Source: CAD feature listing. Evaluate the final solid. Frame: model axes, mm. A direction names the side the tool comes from. Give positions to 0.01 mm unless a question says otherwise; leave off trailing zeros. Loops run counter-clockwise (first coordinate to the right, second up) from the corner with the lowest first, then second, coordinate; pieces in that order, holes last. Notation, with made-up numbers: (-18, -27) -> (34, -27) arc R32 ccw to (34, 9) -> close; hole circle Ø8 at (7.5, 19). An arc over 180 degrees is marked (long way). Return JSON: item names as keys, results as strings. Group by question number.
```python
from build123d import *

# Parameters (mm, degrees)
SKETCH1_R               = 7.5
SKETCH1_R_2             = 2.75
SKETCH1_R_3             = 2.5
BOSS_EXTRUDE1_DEPTH     = 6
CUT_EXTRUDE1_DEPTH      = 70.758959998
CUT_EXTRUDE1_DEPTH_BACK = 70.758959998


with BuildPart() as part:
    # Sketch1 → Boss-Extrude1 (new body)
    # profile 1 of 7: a face of its own
    with BuildSketch(Plane(origin=(0, 0, 0), x_dir=(1, 0, 0), z_dir=(0, 1, 0))):
        with Locations((-52.25, 15.75)):
            Circle(SKETCH1_R)
        with Locations(Location((-52.25, 15.75, 0), (0, 0, 270))):
            Circle(SKETCH1_R_2, mode=Mode.SUBTRACT)
    # profile 2 of 7: a face of its own
    with BuildSketch(Plane(origin=(0, 0, 0), x_dir=(1, 0, 0), z_dir=(0, 1, 0))):
        with BuildLine():
            ThreePointArc((-44.75, 15.75), (-52.25, 8.25), (-59.75, 15.75))
            Line((-59.75, 15.75), (-59.75, -15.75))
            ThreePointArc((-59.75, -15.75), (-52.25, -8.25), (-44.75, -15.75))
            ThreePointArc((-44.75, -15.75), (-48.076702535, -21.981660154), (-55.105623539, -22.685085739))
            Line((-55.105623539, -22.685085739), (-25.355623539, -34.935085739))
            ThreePointArc((-25.355623539, -34.935085739), (-26.673297465, -21.768339846), (-15, -28))
            ThreePointArc((-15, -28), (-17.196699141, -33.303300859), (-22.5, -35.5))
            Line((-22.5, -35.5), (22.5, -35.5))
            ThreePointArc((22.5, -35.5), (17.196699141, -22.696699141), (30, -28))
            Line((30, -28), (30, 28))
            ThreePointArc((30, 28), (17.196699141, 22.696699141), (22.5, 35.5))
            Line((22.5, 35.5), (-22.5, 35.5))
            ThreePointArc((-22.5, 35.5), (-17.196699141, 33.303300859), (-15, 28))
            ThreePointArc((-15, 28), (-26.673297465, 21.768339846), (-25.355623539, 34.935085739))
            Line((-25.355623539, 34.935085739), (-55.105623539, 22.685085739))
            ThreePointArc((-55.105623539, 22.685085739), (-48.076702535, 21.981660154), (-44.75, 15.75))
        make_face()
        with Locations(Location((1.25, -15.75, 0), (0, 0, 270))):
            Circle(SKETCH1_R_2, mode=Mode.SUBTRACT)
        with Locations(Location((1.25, 15.75, 0), (0, 0, 270))):
            Circle(SKETCH1_R_2, mode=Mode.SUBTRACT)
    # profile 3 of 7: a face of its own
    with BuildSketch(Plane(origin=(0, 0, 0), x_dir=(1, 0, 0), z_dir=(0, 1, 0))):
        with Locations((-52.25, -15.75)):
            Circle(SKETCH1_R)
        with Locations(Location((-52.25, -15.75, 0), (0, 0, 270))):
            Circle(SKETCH1_R_2, mode=Mode.SUBTRACT)
    # profile 4 of 7: a face of its own
    with BuildSketch(Plane(origin=(0, 0, 0), x_dir=(1, 0, 0), z_dir=(0, 1, 0))):
        with Locations((-22.5, -28)):
            Circle(SKETCH1_R)
        with Locations(Location((-22.5, -23.5, 0), (0, 0, 270))):
            Circle(SKETCH1_R_3, mode=Mode.SUBTRACT)
    # profile 5 of 7: a face of its own
    with BuildSketch(Plane(origin=(0, 0, 0), x_dir=(1, 0, 0), z_dir=(0, 1, 0))):
        with Locations((22.5, -28)):
            Circle(SKETCH1_R)
        with Locations(Location((22.5, -23.5, 0), (0, 0, 270))):
            Circle(SKETCH1_R_3, mode=Mode.SUBTRACT)
    # profile 6 of 7: a face of its own
    with BuildSketch(Plane(origin=(0, 0, 0), x_dir=(1, 0, 0), z_dir=(0, 1, 0))):
        with Locations((22.5, 28)):
            Circle(SKETCH1_R)
        with Locations(Location((22.5, 23.5, 0), (0, 0, 270))):
            Circle(SKETCH1_R_3, mode=Mode.SUBTRACT)
    # profile 7 of 7: a face of its own
    with BuildSketch(Plane(origin=(0, 0, 0), x_dir=(1, 0, 0), z_dir=(0, 1, 0))):
        with Locations((-22.5, 28)):
            Circle(SKETCH1_R)
        with Locations(Location((-22.5, 23.5, 0), (0, 0, 270))):
            Circle(SKETCH1_R_3, mode=Mode.SUBTRACT)
    extrude(amount=BOSS_EXTRUDE1_DEPTH)

    # Sketch2 → Cut-Extrude1 (cut, two sides: drawn at the far end of the back side and taken through both)
    with BuildSketch(Plane(origin=(0, 6, 0), x_dir=(1, 0, 0), z_dir=(0, 1, 0)).offset(-CUT_EXTRUDE1_DEPTH_BACK)):
        Polygon((-52.25, 11.131197846), (-48.25, 13.440598923), (-48.25, 18.059401077), (-52.25, 20.368802154), (-56.25, 18.059401077), (-56.25, 13.440598923), align=None)
        Polygon((-52.25, -11.131197846), (-56.25, -13.440598923), (-56.25, -18.059401077), (-52.25, -20.368802154), (-48.25, -18.059401077), (-48.25, -13.440598923), align=None)
        Polygon((-2.75, -18.059401077), (1.25, -20.368802154), (5.25, -18.059401077), (5.25, -13.440598923), (1.25, -11.131197846), (-2.75, -13.440598923), align=None)
        Polygon((1.25, 11.131197846), (5.25, 13.440598923), (5.25, 18.059401077), (1.25, 20.368802154), (-2.75, 18.059401077), (-2.75, 13.440598923), align=None)
    extrude(amount=CUT_EXTRUDE1_DEPTH + CUT_EXTRUDE1_DEPTH_BACK, mode=Mode.SUBTRACT)


solid = part.part
```
1) Mould query, pull axis Z, two halves, no side actions, for faces 3 (the face through (-40.022, 2.958, -28.896)), 4 (the face through (5.25, 3, -16)), 5 (the face through (30, 3, 0)). Classes: released by +Z, released by -Z, zero draft, split by the parting line, or undercut.
2) Reachability of faces 1 (the face through (-50.222, 2.958, -19.198)), 2 (the face through (-23.976, 2.958, 35.353)) from +Z, -Z, +X, -X, +Y, -Y: full face, straight path, thin tool, end or side. Return the list, or none.
3) Contact query for a flat-ended pin moving along its axis: P1, Ø1, axis at y = 4, z = -17.5, coming from the -X side. Output: stop coordinate, or through.
4) Cut plane A-A on x = 24. Return loops of the section in (y, z).
5) Cut plane D-D on x = -38. Return loops of the section in (y, z), then the cut area to 3 significant figures.
6) Cut plane C-C on x = -54. Return loops of the section in (y, z), then the cut area to 3 significant figures.
7) Material intervals for line 1 (X direction, y = 1.2, z = 14); line 2 (X direction, y = 2.9, z = 23.5); line 3 (Z direction, x = 20.5, y = 2.9), sorted ascending.
8) Cut plane B-B on y = 2.55. Count the separate pieces of the cut face and the enclosed holes in it, then the cut area to 3 significant figures.
Calculated:
{
 "1": {"face 3": "released by -Z", "face 4": "undercut", "face 5": "zero draft"},
 "2": {"face 1": "+Y, -Y", "face 2": "+Z, -X, +Y, -Y"},
 "3": {"P1": "x = -59.65"},
 "4": {"outline": "(0, -35.35) -> (6, -35.35) -> (6, -25.5) -> (0, -25.5) -> close; (0, -21.5) -> (6, -21.5) -> (6, 21.5) -> (0, 21.5) -> close; (0, 25.5) -> (6, 25.5) -> (6, 35.35) -> (0, 35.35) -> close"},
 "5": {"outline": "(0, -29.73) -> (6, -29.73) -> (6, 29.73) -> (0, 29.73) -> close", "area": "357 mm2"},
 "6": {"outline": "(0, -23.14) -> (6, -23.14) -> (6, -19.36) -> (0, -19.36) -> close; (0, -12.14) -> (6, -12.14) -> (6, 12.14) -> (0, 12.14) -> close; (0, 19.36) -> (6, 19.36) -> (6, 23.14) -> (0, 23.14) -> close", "area": "191 mm2"},
 "7": {"line 1": "-59.75 to -56.25, -48.25 to -2.75, 5.25 to 30", "line 2": "-53.13 to -25, -20 to 20, 25 to 30", "line 3": "-35.5 to -25, -22 to 22, 25 to 35.5"},
 "8": {"separate pieces": "1", "enclosed holes": "8", "area": "5,510 mm2"}
}
